Design review of the part built by this model. Coordinates are the model's own, in mm. Give positions to 0.01 mm unless a question says otherwise; leave off trailing zeros. Order: outer loops, then holes, each group sorted by start corner. A loop starts at its lowest first (then second) coordinate and runs counter-clockwise, first axis right, second up. Notation, with made-up numbers: (70.25, 9.25) -> (79.25, 9.25) arc R17 cw to (79.25, 22.25) -> close; hole circle Ø5 at (39.5, 25.25). An arc over 180 degrees is marked (long way). One line per item, written item: value.
from build123d import *

# Parameters (mm, degrees)
F0_W     = 103.95483
F0_H     = 19.77795
F1_DEPTH = 25
F2_R     = 5.8387
F2_R_2   = 5.669985
F2_R_3   = 5.932122
F2_R_4   = 5.628572
F2_R_5   = 5.846051
F2_R_6   = 5.772215
F2_R_7   = 6.949194
F3_DEPTH = 25
F4_W     = 109.984688
F4_H     = 10.371363
F5_DEPTH = 25


with BuildPart() as f1:
    # F0 (on Top) → F1 (new body)
    with BuildSketch(Plane.XY):
        Rectangle(F0_W, F0_H)
    extrude(amount=F1_DEPTH)

    # F2 (on Top) → F3 (cut)
    with BuildSketch(Plane.XY):
        with Locations((-45.099735, 0)):
            Circle(F2_R)
        with Locations((-32.812502, 0)):
            Circle(F2_R_2)
        with Locations((-19.687502, 0)):
            Circle(F2_R_3)
        with Locations((-7.12101, 0)):
            Circle(F2_R_4)
        with Locations((5.724736, 0)):
            Circle(F2_R_5)
        with Locations((19.128991, 0)):
            Circle(F2_R_6)
        with Locations((33.650268, 0)):
            Circle(F2_R_7)
    extrude(amount=F3_DEPTH, mode=Mode.SUBTRACT)

    # F4 (on Top) → F5 (cut)
    with BuildSketch(Plane.XY):
        with Locations((2.050154, 5.185681)):
            Rectangle(F4_W, F4_H)
    extrude(amount=F5_DEPTH, mode=Mode.SUBTRACT)


solid = f1.part
Item 1: Add section C-C on x = -28.5. Give the boundary of the cut face in (y, z).
Returned:
outline: (-9.89, 0) -> (-3.68, 0) -> (-3.68, 25) -> (-9.89, 25) -> close
Item 2: Add section A-A on z = 6. Give the boundary of the cut face in (x, y).
Returned:
outline: (-51.98, -9.89) -> (51.98, -9.89) -> (51.98, 0) -> (40.6, 0) arc R6.95 cw to (26.7, 0) -> (24.9, 0) arc R5.77 cw to (13.36, 0) -> (11.57, 0) arc R5.85 cw to (-0.12, 0) -> (-1.49, 0) arc R5.63 cw to (-12.75, 0) -> (-13.76, 0) arc R5.93 cw to (-25.62, 0) -> (-27.14, 0) arc R5.67 cw to (-38.48, 0) -> (-39.26, 0) arc R5.84 cw to (-50.94, 0) -> (-51.98, 0) -> close
Item 3: Add section D-D on x = -4. Give the boundary of the cut face in (y, z), plus the area to 3 significant figures.
Returned:
outline: (-9.89, 0) -> (-4.68, 0) -> (-4.68, 25) -> (-9.89, 25) -> close
area: 130 mm²
Item 4: To check wall thickness, follow line 1 along Y through (x, z) = (19.5, 16); line 2 along X through (y, z) = (-6.25, 22.25); line 3 along Y through (x, z) = (31.5, 1.5). State the ranges of each line that lie inside material, in increasing order. Write a range as from..to.
Returned:
line 1: -9.89..-5.76
line 2: -51.98..30.61, 36.69..51.98
line 3: -9.89..-6.61
Item 5: Add section B-B on y = -4.75. Count the separate pieces of the cut face and the enclosed holes in it, plus the area to 3 significant figures.
Returned:
separate pieces: 8
enclosed holes: 0
area: 1,360 mm²
Item 6: Draft analysis for pull direction X (two halves, no side actions). For faces 1 (the flat face through (51.977, -5, 12)), 2 (the flat face through (26, 0, 12)), 3 (the cylindrical face through (5.596, -5.845, 12.325)), state which applies: pulls with the +X half, pulls with the -X half, needs draft (parallel to the pull), parting line crosses it, or undercut.
Returned:
face 1: pulls with the +X half
face 2: needs draft
face 3: undercut
